CAD build for the part. Positions are in the model's coordinates, mm. A direction names the side the tool comes from. Coordinates: 2 decimals unless noted, no trailing zeros. Loops run counter-clockwise (first coordinate to the right, second up) from the corner with the lowest first, then second, coordinate; pieces in that order, holes last. Notation, with made-up numbers: M 51.25,-24.5 L 59.25,-24.5 A12 ccw 59.25,-16.5 Z; hole C -5.75,-37 d2. An arc over 180 degrees is marked long. Answer as a JSON object with one key per item and string values. Group by question number.
Autodesk Inventor part; units mm, degrees
ref_plane "YZ Plane" through (0, 0, 0) normal (1, 0, 0) x (0, 1, 0)
ref_plane "XZ Plane" through (0, 0, 0) normal (0, 1, 0) x (-1, 0, 0)
ref_plane "XY Plane" through (0, 0, 0) normal (0, 0, 1) x (1, 0, 0)
sketch "Boceto1" plane through (0, 0, 0) normal (0, 0, 1) x (1, 0, 0)
  line L0 (0, 0) -> (24.2042, 0) construction
  line L1 (0, 9.5) -> (11, 9.5)
  line L2 (0, 9.5) -> (0, 50)
  line L3 (0, 50) -> (4, 50)
  line L4 (4, 50) -> (4, 20)
  line L5 (4, 20) -> (20, 20)
  line L6 (20, 20) -> (20, 13.925)
  line L7 (20, 13.925) -> (11, 13.925)
  line L8 (11, 13.925) -> (11, 9.5)
  line L9 (0, 0) -> (0, 63.5344) construction
  line L10 (10.3397, 15) -> (10.3397, 20) construction
  line L11 (10.3397, 20) -> (20, 20) construction
  dimension "d0" = 50
  dimension "d1" = 4
  dimension "d4" = 13.925
  dimension "d10" = 9.5
  dimension "d11" = 9
  dimension "d13" = 20
  dimension "d15" = 20
revolve "Revolución1" add sketch "Boceto1" angle 360 about axis through (0, 0, 0) along (1, 0, 0)
sketch "Sketch2" plane through (20, 0, 0) normal (1, 0, 0) x (0, 0, -1)
  circle A0 centre (0, 0) radius 13
  circle A1 centre (0, 0) radius 13.925
  dimension "d16" = 26
extrude "Extrusion1" add sketch "Sketch2" against normal up to surface (9 mm away)
properties part number "Reel1ACABARMEDIDAS"
Item 1: Slice it at C-C, the plane x = 2.25. Write the cut outline in (y, z).
Item 2: Drill centre lines: L1, parallel to Z at x = 5.5, y = 0; L2, parallel to Z at x = 2.5, y = 0; L3, parallel to X at y = 22.5, z = -39.5. Where is each one in solid material? Low to high. Write a range as from..to.
Item 3: Tool access for faces 4 (the cylindrical face through (15.563, -7.91, 10.316)), 5 (the flat face through (20, -4, -13)): list every direction of +Z, -Z, +X, -X, +Y, -Y with a clear straight run to the whole face (end or side of a thin tool).
Item 4: Slice it at D-D, the plane z = -15. Write the cut outline in (x, y).
Item 5: Pull direction Z, two halves, no side cores. Call faces 1 (the flat face through (4, -1, -22)), 2 (the cylindrical face through (12.112, -4.336, -19.524)), 3 (the cylindrical face through (5.58, 4.38, -8.43)): released by +Z, released by -Z, zero draft, split by the parting line, or undercut.
Item 6: Slice it at A-A, the plane y = 0. Write the cut outline in (x, z), then the cut area to 3 significant figures.
Item 7: Pin check, flat tips, straight feed: pin 1 (8 mm diameter, centred on x = 13, z = -16, fed in from -Y); pin 2 (1 mm diameter, centred on y = -30.5, z = 8, fed in from -X); pin 3 (8 mm diameter, centred on x = 10, y = -10.5, fed in from +Z); pin 4 (1.5 mm diameter, centred on x = 8, z = 7.5, fed in from -Y). Stop position of each tip, or through.
Computed:
{
 "1": {"outline": "C 0,0 d100; hole C 0,0 d19"},
 "2": {"L1": "-20..-9.5, 9.5..20", "L2": "-50..-9.5, 9.5..50", "L3": "0..4"},
 "3": {"face 4": "+X", "face 5": "+Z, -Z, +X, +Y, -Y"},
 "4": {"outline": "M 0,-47.7 L 4,-47.7 L 4,-13.23 L 20,-13.23 L 20,13.23 L 4,13.23 L 4,47.7 L 0,47.7 Z"},
 "5": {"face 1": "zero draft", "face 2": "split by the parting line", "face 3": "undercut"},
 "6": {"outline": "M 0,-50 L 4,-50 L 4,-20 L 20,-20 L 20,-13 L 11,-13 L 11,-9.5 L 0,-9.5 Z; M 0,9.5 L 11,9.5 L 11,13 L 20,13 L 20,20 L 4,20 L 4,50 L 0,50 Z", "area": "597 mm2"},
 "7": {"pin 1": "y = -16", "pin 2": "x = 0", "pin 3": "z = 18.91", "pin 4": "y = -18.83"}
}
